Check sheet for the modelled part. Datum: model origin and axes. Units: mm. Give positions to 0.01 mm unless a question says otherwise; leave off trailing zeros. Loops run counter-clockwise (first coordinate to the right, second up) from the corner with the lowest first, then second, coordinate; pieces in that order, holes last. Notation, with made-up numbers: (30, 10) -> (87, 10) arc R21 ccw to (87, 15) -> close; hole circle Ø3 at (-40, -1). An arc over 180 degrees is marked (long way). Write each question's results on one line, items separated by ' | '. Start each with the question number.
Item 1: Gauge pin test, flat end, axial feed: pin 1 Ø3.5 at (x, y) = (-15.25, 15.25) entering from +Z. Record the tip position at first contact, or that the pin passes through.
Item 2: Scan lines: line 1 along X through (y, z) = (24.5, 1.4); line 2 along Y through (x, z) = (-15, 1.85); line 3 along Y through (x, z) = (-17, 0.35). Record each from-to range of solid material in increasing order.
Item 3: Cross-section at A-A on x = -19. Enter the section's corners in (y, z).
Item 4: Cross-section at D-D on y = -25. Enter the section's corners in (x, z), then the cut area to 3 significant figures.
Item 5: Cross-section at B-B on y = -2.5. Enter the section's corners in (x, z).
Item 6: Cross-section at C-C on y = 21. Enter the section's corners in (x, z).
from build123d import *

# Parameters (mm, degrees)
F0_R     = 2.3
F1_DEPTH = 2
F4_R     = 7.99999
F5_R     = 2.4


# Not quite as in the source:
# - a fillet or chamfer is up to 0.001 mm smaller than in the source, because OpenCascade refuses the exact size


with BuildPart() as f1:
    # F0 (on Top) → F1 (new body)
    with BuildSketch(Plane.XY):
        Polygon((12.313708499, 1), (36.9456929209, 25.6319844219), (31.2888386714, 31.2888386714), (25.6319844219, 36.9456929209), (1, 12.313708499), (0, 11.313708499), (0, 0), (11.313708499, 0), align=None)
        with Locations((3.9999969952, 3.9999969952)):
            Circle(F0_R, mode=Mode.SUBTRACT)
        with Locations((15.2499951732, 15.2499951732)):
            Circle(F0_R, mode=Mode.SUBTRACT)
        with Locations((26.4999933512, 26.4999933512)):
            Circle(F0_R, mode=Mode.SUBTRACT)
        Polygon((0, 11.313708499), (1, 12.313708499), (0, 12.313708499), align=None)
        Polygon((12.313708499, 0), (12.313708499, 1), (11.313708499, 0), align=None)
    extrude(amount=F1_DEPTH)

    # F2: F1 across plane


with BuildPart() as f1_1:
    add(f1.part)
    add(f1.part.mirror(Plane.YZ))

    # F3: F1 across plane


with BuildPart() as f1_2:
    add(f1_1.part)
    add(f1_1.part.mirror(Plane.XZ))

    # F4 (radius 8 in the source; OpenCascade refuses exactly that, so slightly less here)
    f4_edges = [f1_2.edges().sort_by_distance(p)[0] for p in [
        (-25.631984, 36.945693, 1),
        (-36.945693, 25.631984, 1),
        (-36.945693, -25.631984, 1),
        (-25.631984, -36.945693, 1),
        (25.631984, -36.945693, 1),
        (36.945693, -25.631984, 1),
        (36.945693, 25.631984, 1),
        (25.631984, 36.945693, 1),
    ]]
    fillet(f4_edges, radius=F4_R)

    # F5
    f5_edges = [f1_2.edges().sort_by_distance(p)[0] for p in [
        (12.313708, 1, 1),
        (12.313708, -1, 1),
        (1, 12.313708, 1),
        (-1, 12.313708, 1),
        (-12.313708, 1, 1),
        (-12.313708, -1, 1),
        (-1, -12.313708, 1),
        (1, -12.313708, 1),
    ]]
    fillet(f5_edges, radius=F5_R)


solid = f1_2.part
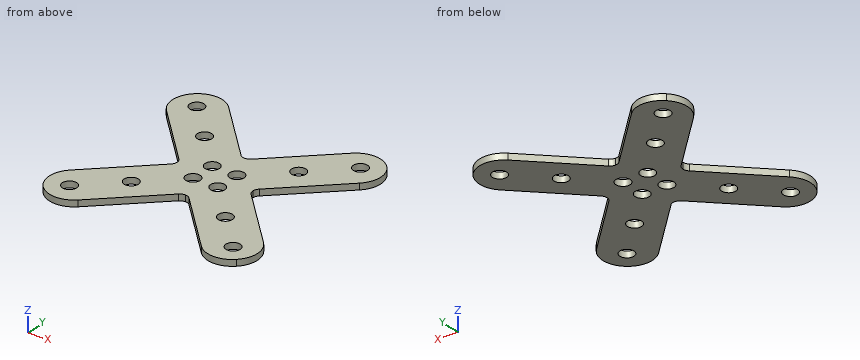
Answer sheet:
1) pin 1: passes through
2) line 1: x = -33.55 to -27.64, -25.36 to -13.19, 13.19 to 25.36, 27.64 to 33.55 | line 2: y = -26.31 to -17.54, -12.96 to -3.69, 3.69 to 12.96, 17.54 to 26.31 | line 3: y = -28.31 to -16.74, -13.76 to -5.69, 5.69 to 13.76, 16.74 to 28.31
3) outline: (-30.31, 0) -> (-7.69, 0) -> (-7.69, 2) -> (-30.31, 2) -> close; (7.69, 0) -> (30.31, 0) -> (30.31, 2) -> (7.69, 2) -> close
4) outline: (-33.61, 0) -> (-28.24, 0) -> (-28.24, 2) -> (-33.61, 2) -> close; (-24.76, 0) -> (-13.69, 0) -> (-13.69, 2) -> (-24.76, 2) -> close; (13.69, 0) -> (24.76, 0) -> (24.76, 2) -> (13.69, 2) -> close; (28.24, 0) -> (33.61, 0) -> (33.61, 2) -> (28.24, 2) -> close | area: 65.7 mm²
5) outline: (-13.81, 0) -> (-5.74, 0) -> (-5.74, 2) -> (-13.81, 2) -> close; (-2.26, 0) -> (2.26, 0) -> (2.26, 2) -> (-2.26, 2) -> close; (5.74, 0) -> (13.81, 0) -> (13.81, 2) -> (5.74, 2) -> close
6) outline: (-32.15, 0) -> (-9.69, 0) -> (-9.69, 2) -> (-32.15, 2) -> close; (9.69, 0) -> (32.15, 0) -> (32.15, 2) -> (9.69, 2) -> close
